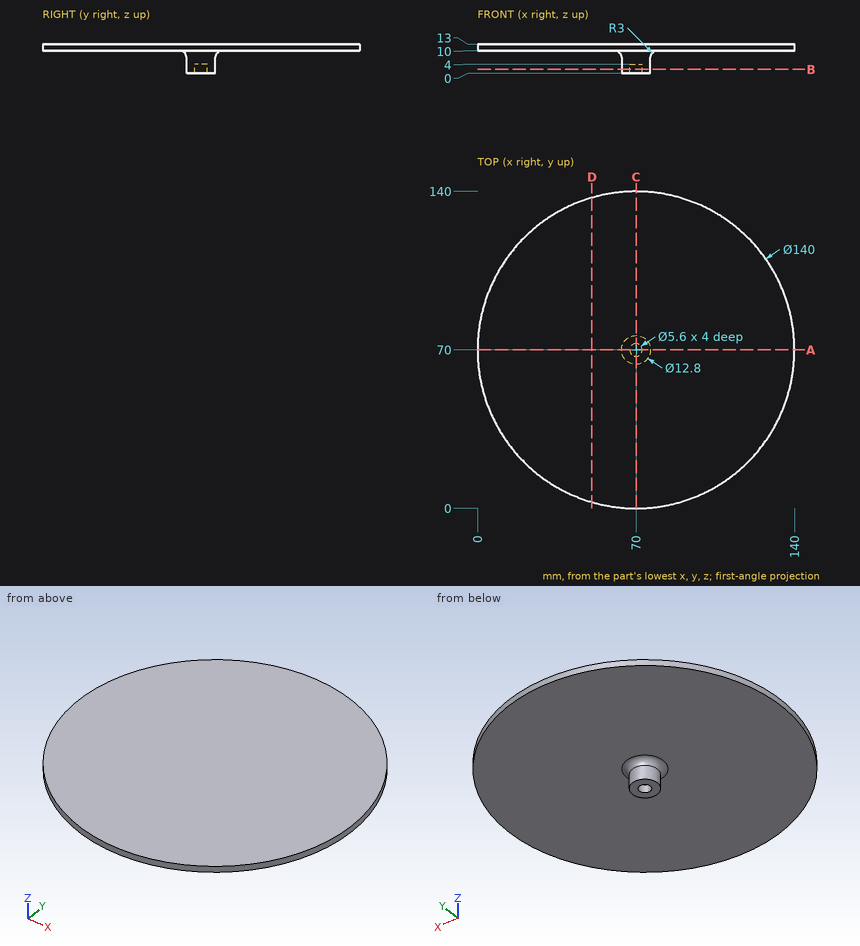
The figure shows three views and two pictorial views of one solid part (mm, origin at its lowest corner). Answer the questions. Coordinates: 2 decimals unless noted, no trailing zeros. Write each loop counter-clockwise with the first axis right and the second up, starting at its lowest first coordinate (ties: lowest second). Pieces come first, ordered by that corner, then holes.
1. The part is cut by section A-A, the plane y = 70. Write down the section's boundary in (x, z), and give its area (3 significant figures).
Results list:
outline: (0, 10) - (60.6, 10) arc R3 cw to (63.6, 7) - (63.6, 0) - (67.2, 0) - (67.2, 4) - (72.8, 4) - (72.8, 0) - (76.4, 0) - (76.4, 7) arc R3 cw to (79.4, 10) - (140, 10) - (140, 13) - (0, 13) - close
area: 529 mm2
2. Consider line 1 along Y through (x, z) = (70, 1.8); line 2 along Z through (x, y) = (76, 92.5); line 3 along Y through (x, z) = (70.5, 5.5). Determine where each line is inside the solid, lowest interval first.
Results list:
line 1: y = 63.6 to 67.2, 72.8 to 76.4
line 2: z = 10 to 13
line 3: y = 63.62 to 76.38
3. The part is cut by section D-D, the plane x = 50.5. Write down the section's boundary in (y, z).
Results list:
outline: (2.77, 10) - (137.23, 10) - (137.23, 13) - (2.77, 13) - close
4. The part is cut by section B-B, the plane z = 1.75. Write down the section's boundary in (x, y), and give its area (3 significant figures).
Results list:
outline: circle Ø12.8 at (70, 70); hole circle Ø5.6 at (70, 70)
area: 104 mm2
5. A flat-ended cylindrical pin translates along its axis: pin 1 (6 mm diameter, centred on x = 69.5, y = 69.5, fed in from -Z). Find the tip coordinate at first contact, or state that the pin passes through.
Results list:
pin 1: stops at z = 0
